```python
from build123d import *

# Parameters (mm, degrees)
SKETCH1_W           = 40
SKETCH1_H           = 7.5
BOSS_EXTRUDE1_DEPTH = 80
SHELL1_T            = -4
FILLET1_R           = 3
SKETCH2_W           = 32
SKETCH2_H           = 72
BOSS_EXTRUDE2_DEPTH = 2


with BuildPart() as part:
    # Sketch1 → Boss-Extrude1 (new body)
    with BuildSketch(Plane.XY):
        with Locations((20, 3.75)):
            Rectangle(SKETCH1_W, SKETCH1_H)
    extrude(amount=BOSS_EXTRUDE1_DEPTH)

    # Shell1
    shell1_openings = [part.faces().sort_by_distance(p)[0] for p in [
        (20, 7.5, 40),
    ]]
    offset(amount=SHELL1_T, openings=shell1_openings, kind=Kind.INTERSECTION)

    # Fillet1
    fillet1_edges = [part.edges().sort_by_distance(p)[0] for p in [
        (40, 3.75, 80),
        (0, 3.75, 80),
        (40, 3.75, 0),
        (20, 0, 0),
        (0, 3.75, 0),
        (40, 0, 40),
        (0, 0, 40),
        (20, 0, 80),
    ]]
    fillet(fillet1_edges, radius=FILLET1_R)

    # Sketch2 → Boss-Extrude2 (add)
    with BuildSketch(Plane(origin=(0, 7.5, 0), x_dir=(1, 0, 0), z_dir=(0, 1, 0))):
        with BuildLine():
            Line((3.65, -77.85), (36.35, -77.85))
            ThreePointArc((36.35, -77.85), (37.410660172, -77.410660172), (37.85, -76.35))
            Line((37.85, -76.35), (37.85, -3.65))
            ThreePointArc((37.85, -3.65), (37.410660172, -2.589339828), (36.35, -2.15))
            Line((36.35, -2.15), (3.65, -2.15))
            ThreePointArc((3.65, -2.15), (2.589339828, -2.589339828), (2.15, -3.65))
            Line((2.15, -3.65), (2.15, -76.35))
            ThreePointArc((2.15, -76.35), (2.589339828, -77.410660172), (3.65, -77.85))
        make_face()
        with Locations((20, -40)):
            Rectangle(SKETCH2_W, SKETCH2_H, mode=Mode.SUBTRACT)
    extrude(amount=BOSS_EXTRUDE2_DEPTH)


solid = part.part
```
Input: part model. Units: mm. Frame: model coordinates. A direction names the side the tool comes from. Give positions to 0.01 mm unless a question says otherwise; leave off trailing zeros. Order: outer loops, then holes, each group sorted by start corner. A loop starts at its lowest first (then second) coordinate and runs counter-clockwise, first axis right, second up. Notation, with made-up numbers: (11.25, 80.25) -> (61.25, 80.25) arc R30 ccw to (61.25, 113.25) -> close; hole circle Ø10 at (45.25, 62). An arc over 180 degrees is marked (long way). Write each question's results on one line, items separated by ' | '. Start each with the question number.
Item 1: Line query: line 1 (Z direction, x = 4.5, y = 7); line 2 (X direction, y = 8, z = 52); line 3 (Z direction, x = 25, y = 8.5). Output: solid intervals per line, ascending.
Item 2: Contact query for flat-ended pins moving along their axis: P1, Ø9.5, axis at x = 19, z = 43, coming from the +Y side; P2, Ø0.6, axis at y = 9, z = 35, coming from the +X side; P3, Ø2, axis at y = 9, z = 26, coming from the -X side. Output: stop coordinate, or through.
Item 3: Set-up query: faces 1 (the flat face through (20, 8, 2.15)), 2 (the cylindrical face through (2.58, 8.49, 77.4)), 3 (the flat face through (36, 7, 41)). Return all of +Z, -Z, +X, -X, +Y, -Y with unobstructed straight access to the full face (end or side cutting, diameter ignored); none if empty.
Item 4: Cut plane B-B on x = 17.5. Return the cut outline in (y, z), then the cut area to 3 significant figures.
Item 5: Cut plane C-C on y = 1.5. Return the cut outline in (x, z).
Item 6: Mould query, pull axis X, two halves, no side actions, for faces 4 (the flat face through (20, 7, 4)), 5 (the flat face through (20, 5, 80)), 6 (the flat face through (0, 5, 39)). Classes: pulls with the +X half, pulls with the -X half, needs draft (parallel to the pull), parting line crosses it, or undercut.
Item 7: Cut plane A-A on z = 63.5. Return the cut outline in (x, y), then the cut area to 3 significant figures.
Established:
1) line 1: 0 to 4, 76 to 80 | line 2: 2.15 to 4, 36 to 37.85 | line 3: 2.15 to 4, 76 to 77.85
2) P1: y = 4 | P2: x = 37.85 | P3: x = 2.15
3) face 1: -Z, +X, -X, +Y | face 2: +Z, -X, +Y | face 3: +Y
4) outline: (0, 3) arc R3 ccw to (3, 0) -> (7.5, 0) -> (7.5, 2.15) -> (9.5, 2.15) -> (9.5, 4) -> (4, 4) -> (4, 76) -> (9.5, 76) -> (9.5, 77.85) -> (7.5, 77.85) -> (7.5, 80) -> (3, 80) arc R3 ccw to (0, 77) -> close | area: 352 mm^2
5) outline: (0.4, 3) arc R2.6 ccw to (3, 0.4) -> (37, 0.4) arc R2.6 ccw to (39.6, 3) -> (39.6, 77) arc R2.6 ccw to (37, 79.6) -> (3, 79.6) arc R2.6 ccw to (0.4, 77) -> close
6) face 4: undercut | face 5: needs draft | face 6: pulls with the -X half
7) outline: (0, 3) arc R3 ccw to (3, 0) -> (37, 0) arc R3 ccw to (40, 3) -> (40, 7.5) -> (37.85, 7.5) -> (37.85, 9.5) -> (36, 9.5) -> (36, 4) -> (4, 4) -> (4, 9.5) -> (2.15, 9.5) -> (2.15, 7.5) -> (0, 7.5) -> close | area: 192 mm^2
